Verification items for the finished model (mm, model axes). Face numbers are marked on the shaded views. A direction names the side the tool comes from. Round coordinates to 2 decimals unless told otherwise and drop trailing zeros. Write each loop counter-clockwise with the first axis right and the second up, starting at its lowest first coordinate (ties: lowest second). Pieces come first, ordered by that corner, then holes. Notation, with made-up numbers: M 40,-30.75 L 89,-30.75 A16 cw 89,-23.75 Z; hole C 32,52.25 d3. An arc over 180 degrees is marked long. Write each question's results on one line, items separated by ' | '.
from build123d import *

# Parameters (mm, degrees)
SKETCH1_W           = 6
SKETCH1_H           = 6
BOSS_EXTRUDE1_DEPTH = 8.31
SKETCH2_R           = 2.125
CUT_EXTRUDE1_DEPTH  = 10
SKETCH3_R           = 3.75
BOSS_EXTRUDE2_DEPTH = 55


with BuildPart() as part:
    # Sketch1 → Boss-Extrude1 (new body)
    with BuildSketch(Plane(origin=(0, 0, 0), x_dir=(1, 0, 0), z_dir=(0, 1, 0))):
        with Locations((3, 3)):
            Rectangle(SKETCH1_W, SKETCH1_H)
    extrude(amount=BOSS_EXTRUDE1_DEPTH)

    # Sketch2 → Cut-Extrude1 (cut)
    with BuildSketch(Plane(origin=(6, 0, 0), x_dir=(0, 0, -1), z_dir=(1, 0, 0))):
        with Locations((3, 3.31)):
            Circle(SKETCH2_R)
    extrude(amount=-CUT_EXTRUDE1_DEPTH, mode=Mode.SUBTRACT)

    # Sketch3 → Boss-Extrude2 (add)
    with BuildSketch(Plane(origin=(0, 8.31, 0), x_dir=(1, 0, 0), z_dir=(0, 1, 0))):
        with Locations((3, 3)):
            Circle(SKETCH3_R)
    extrude(amount=BOSS_EXTRUDE2_DEPTH)


solid = part.part
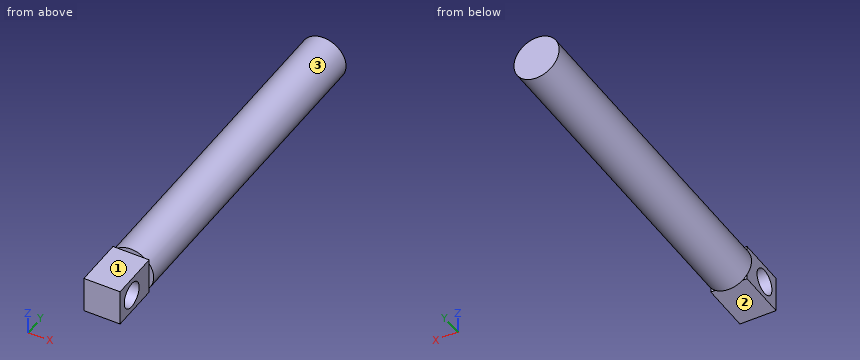
1) Sectioned sample at A-A, the plane y = 3.31. Record the cut outline in (x, z) (3 decimals), and give its area (3 significant figures).
Calculated:
outline: M 0,-6 L 6,-6 L 6,-5.125 L 0,-5.125 Z; M 0,-0.875 L 6,-0.875 L 6,0 L 0,0 Z | area: 10.5 mm²
2) Sectioned sample at C-C, the plane x = 3. Record the cut outline in (y, z) (3 decimals).
Calculated:
outline: M 0,-6 L 8.31,-6 L 8.31,-6.75 L 63.31,-6.75 L 63.31,0.75 L 8.31,0.75 L 8.31,0 L 0,0 Z; hole C 3.31,-3 d4.25
3) Depth check by flat-ended pin: P1, Ø1.8, axis at y = 4, z = -2.5, coming from the -X side; P2, Ø0.8, axis at x = 6.5, z = -2.5, coming from the -Y side; P3, Ø3, axis at x = 4.5, y = 6, coming from the +Z side. Enter the tip coordinate at first touch or a pass-through.
Calculated:
P1: passes through | P2: stops at y = 8.31 | P3: stops at z = 0
4) Sectioned sample at D-D, the plane y = 23.5. Record the cut outline in (x, z).
Calculated:
outline: C 3,-3 d7.5
5) Material ranges on line 1 (Y direction, x = 4.2, z = -3) (3 decimals); line 2 (X direction, y = 55, z = -2.75); line 3 (X direction, y = 38.5, z = -6), recorded low to high. Write a range as [from, to].
Calculated:
line 1: y = [0, 1.185], [5.435, 63.31] | line 2: x = [-0.74, 6.74] | line 3: x = [0.75, 5.25]
6) Sectioned sample at B-B, the plane z = -3. Record the cut outline in (x, y) (3 decimals), and give its area (3 significant figures).
Calculated:
outline: M -0.75,8.31 L 0,8.31 L 0,5.435 L 6,5.435 L 6,8.31 L 6.75,8.31 L 6.75,63.31 L -0.75,63.31 Z; M 0,0 L 6,0 L 6,1.185 L 0,1.185 Z | area: 437 mm²
7) Access from +Z, -Z, +X, -X, +Y, -Y to the whole of each face (thin tool, end or side, straight path). Record for the marked faces 1, 2 and 3.
Calculated:
face 1: +Z, +X, -X, -Y | face 2: -Z, +X, -X, -Y | face 3: +Y
